```python
from build123d import *

# Parameters (mm, degrees)
BOSS_EXTRUDE1_DEPTH = 150
SKETCH2_W           = 60
SKETCH2_H           = 60
SKETCH2_R           = 15
BOSS_EXTRUDE2_DEPTH = 76
FILLET1_R           = 30
RIB4_REACH          = 181.042
SKETCH5_WALL_W      = 480.08378995
SKETCH5_WALL_H      = 12


with BuildPart() as part:
    # Sketch1 → Boss-Extrude1 (new body)
    with BuildSketch(Plane(origin=(0, 0, 0), x_dir=(1, 0, 0), z_dir=(0, 1, 0))):
        Polygon((0, 50), (0, 26), (10, 26), (10, -26), (0, -26), (0, -50), (12, -50), (12, -38), (24, -38), (24, 38), (12, 38), (12, 50), align=None)
    extrude(amount=BOSS_EXTRUDE1_DEPTH)

    # Sketch2 → Boss-Extrude2 (add)
    with BuildSketch(Plane(origin=(0, 0, -38), x_dir=(-1, 0, 0), z_dir=(0, 0, -1))):
        with Locations((-54, 120)):
            Rectangle(SKETCH2_W, SKETCH2_H)
        with Locations((-54, 120)):
            Circle(SKETCH2_R, mode=Mode.SUBTRACT)
    extrude(amount=-BOSS_EXTRUDE2_DEPTH)

    # Fillet1
    fillet1_edges = [part.edges().sort_by_distance(p)[0] for p in [
        (84, 150, 0),
        (84, 90, 0),
    ]]
    fillet(fillet1_edges, radius=FILLET1_R - 0.0001)  # a hair under: the kernel refuses the full size

    # Sketch5 wall → Rib4 (add, up to next)
    with BuildSketch(Plane(origin=(52.235294323, 52.941176856, 0), x_dir=(0.470588235292, 0.882352941178, 0), z_dir=(-0.882352941178, 0.470588235292, 0)), mode=Mode.PRIVATE) as rib4_sk1:
        Rectangle(SKETCH5_WALL_W, SKETCH5_WALL_H)
    rib4_tool1 = extrude(rib4_sk1.sketch, amount=RIB4_REACH, mode=Mode.PRIVATE) - part.part
    add(rib4_tool1.solids().sort_by_distance((52.235294323, 52.941176856, 0))[0])


solid = part.part
```
The model under review builds one solid part; all positions refer to its coordinate system, in mm. A direction names the side the tool comes from. Round coordinates to 2 decimals unless told otherwise and drop trailing zeros. Loops run counter-clockwise (first coordinate to the right, second up) from the corner with the lowest first, then second, coordinate; pieces in that order, holes last. Notation, with made-up numbers: (52, 85.25) - (74, 85.25) arc R19 cw to (74, 108.25) - close; hole circle Ø7 at (62.25, 1.25). An arc over 180 degrees is marked (long way). Use a Markdown table: item, result. Add a question column.
Q1. The part is to be moulded in two halves that separate along Z. For faces 1 (the face through (5, 74, -26)), 2 (the face through (24, 44, 22)), 3 (the face through (41, 109, 38)), 4 (the face through (10, 74, 0)), say which applies: pulls with the +Z half, pulls with the -Z half, needs draft (parallel to the pull), parting line crosses it, or undercut.
Q2. Add section B-B (x = 59.5). State the section outline as (y, z) points.
Q3. Machinability: for faces 5 (the face through (39, 90, -22)), 6 (the face through (12, 74, -44)), 7 (the face through (75.445, 99.021, 8.976)), which of the approach directions +Z, -Z, +X, -X, +Y, -Y give a long, thin tool a straight path to every point of the face, cutting with its end or side? Answer none if there is none.
Q4. Insertion check: pin 1 Ø6 at (y, z) = (90.5, 24.5) entering from +X; pin 2 Ø21.5 at (x, y) = (38.5, 101) entering from -Z; pin 3 Ø1.5 at (x, z) = (44.5, 15) entering from -Y. Each pin has a flat end and moves straight along its axis. Give the tip position at first contact, or say it passes through.
Q5. Add section D-D (y = 63.5). State the section outline as (x, z) points.
Q6. Add section C-C (y = 110). State the section outline as (x, z) points, plus the area to 3 significant figures.
Q7. For probe 1 along Y at (x, z) = (54, 19); probe 2 along Z at (x, y) = (9, 68); probe 3 along X at (y, z) = (81.5, 25.5), list the stretches that pass through material, from the lowest coordinate up.
Worked answers:
| question | item | result |
|---|---|---|
| 1 | face 1 | undercut |
| 1 | face 2 | needs draft |
| 1 | face 3 | pulls with the +Z half |
| 1 | face 4 | undercut |
| 2 | outline | (66.56, -6) - (90.51, -6) - (90.51, -38) - (106.04, -38) - (106.04, 38) - (90.51, 38) - (90.51, 6) - (66.56, 6) - close; (133.96, -38) - (149.49, -38) - (149.49, 38) - (133.96, 38) - close |
| 3 | face 5 | -Z, +X, -Y |
| 3 | face 6 | -Z, +X, +Y, -Y |
| 3 | face 7 | +X, -Y |
| 4 | pin 1 | x = 68.06 |
| 4 | pin 2 | z = -38 |
| 4 | pin 3 | y = 90 |
| 5 | outline | (0, -50) - (12, -50) - (12, -38) - (24, -38) - (24, -6) - (57.87, -6) - (57.87, 6) - (24, 6) - (24, 38) - (12, 38) - (12, 50) - (0, 50) - (0, 26) - (10, 26) - (10, -26) - (0, -26) - close |
| 6 | outline | (0, -50) - (12, -50) - (12, -38) - (42.82, -38) - (42.82, 38) - (12, 38) - (12, 50) - (0, 50) - (0, 26) - (10, 26) - (10, -26) - (0, -26) - close; (65.18, -38) - (82.28, -38) - (82.28, 38) - (65.18, 38) - close |
| 6 | area | 4,320 mm² |
| 7 | probe 1 | 90 to 105, 135 to 150 |
| 7 | probe 2 | -50 to -26, 26 to 50 |
| 7 | probe 3 | 10 to 24 |
